Can you work these out from the drawing? Everything is in mm from the part's minimum corner. A direction names the side the tool comes from. Round coordinates to 2 decimals unless told otherwise and drop trailing zeros. Loops run counter-clockwise (first coordinate to the right, second up) from the corner with the lowest first, then second, coordinate; pieces in that order, holes last. Notation, with made-up numbers: (-24.5, 22.5) -> (-13.5, 22.5) arc R16 ccw to (-13.5, 34.5) -> close; hole circle Ø4 at (68, 52). An arc over 180 degrees is marked (long way). One line per item, written item: value.
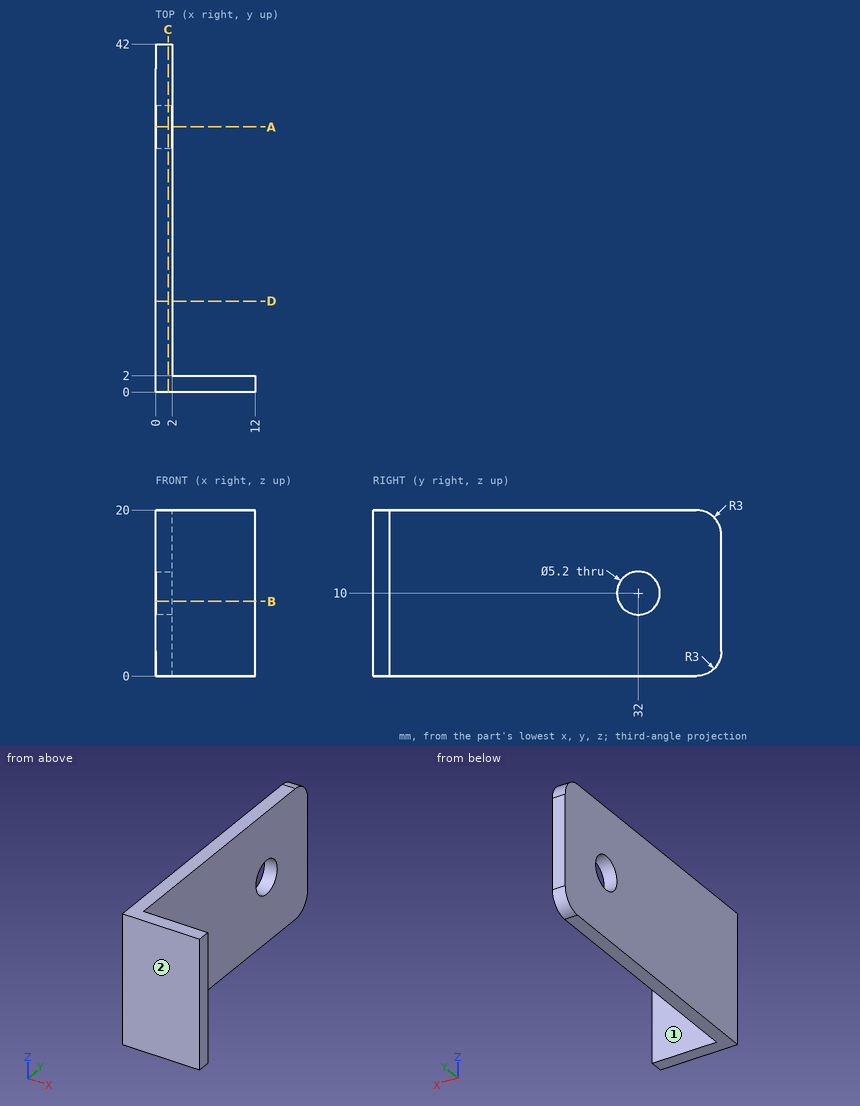
Item 1: If we section it at C-C on x = 1.5: List the corners of the cut face in (y, z) for me, plus the area to 3 significant figures.
Output:
outline: (0, 0) -> (39, 0) arc R3 ccw to (42, 3) -> (42, 17) arc R3 ccw to (39, 20) -> (0, 20) -> close; hole circle Ø5.2 at (32, 10)
area: 815 mm²
Item 2: If we section it at A-A on y = 32: List the corners of the cut face in (x, z) for me.
Output:
outline: (0, 0) -> (2, 0) -> (2, 7.4) -> (0, 7.4) -> close; (0, 12.6) -> (2, 12.6) -> (2, 20) -> (0, 20) -> close
Item 3: I need wall thicknesses on line 1 (Y direction, x = 1.2, z = 10); line 2 (X direction, y = 16, z = 14.5). Which ranges of each line are inside material? Lowest first, please. Write a range as from..to.
Output:
line 1: y = 0..29.4, 34.6..42
line 2: x = 0..2
Item 4: If we section it at D-D on y = 11: List the corners of the cut face in (x, z) for me.
Output:
outline: (0, 0) -> (2, 0) -> (2, 20) -> (0, 20) -> close
Item 5: If we section it at B-B on z = 9: List the corners of the cut face in (x, y) for me.
Output:
outline: (0, 0) -> (12, 0) -> (12, 2) -> (2, 2) -> (2, 29.6) -> (0, 29.6) -> close; (0, 34.4) -> (2, 34.4) -> (2, 42) -> (0, 42) -> close
Item 6: Will these pins go through, and if not, where does the flat tip stop? pin 1 Ø4 at (x, y) = (4.5, 32) entering from +Z; pin 2 Ø3 at (x, z) = (5.5, 7) entering from +Y; pin 3 Ø2 at (y, z) = (22, 17.5) entering from +X.
Output:
pin 1: passes through
pin 2: stops at y = 2
pin 3: stops at x = 2
Item 7: For the marked faces 1 and 2, which set-ups out of +Z, -Z, +X, -X, +Y, -Y let a thin tool reach every point of the face, with its end or its side?
Output:
face 1: +Z, -Z, +X, +Y
face 2: +Z, -Z, +X, -X, -Y
